```python
from build123d import *

# Parameters (mm, degrees)
SKETCH1_R           = 12.85
BOSS_EXTRUDE5_DEPTH = 10.58
SKETCH4_R           = 7.5
SKETCH4_R_2         = 4.5
BOSS_EXTRUDE6_DEPTH = 10.58


with BuildPart() as part:
    # Sketch1 → Boss-Extrude5 (new body)
    with BuildSketch(Plane.XY):
        Circle(SKETCH1_R)
    extrude(amount=BOSS_EXTRUDE5_DEPTH)

    # Sketch4 → Boss-Extrude6 (add)
    with BuildSketch(Plane(origin=(0, 0, 0), x_dir=(1, 0, 0), z_dir=(0, 1, 0))):
        with BuildLine():
            Line((-7.5, -10.58), (-7.5, -23.749253103))
            ThreePointArc((-7.5, -23.749253103), (0, -16.249253103), (7.5, -23.749253103))
            Line((7.5, -23.749253103), (7.5, -10.58))
            Line((7.5, -10.58), (-7.5, -10.58))
        make_face()
        with Locations((0, -23.749253103)):
            Circle(SKETCH4_R)
        with Locations((0, -23.749253103)):
            Circle(SKETCH4_R_2, mode=Mode.SUBTRACT)
        with Locations((0, -23.749253103)):
            Circle(SKETCH4_R_2)
    extrude(amount=BOSS_EXTRUDE6_DEPTH)


solid = part.part
```
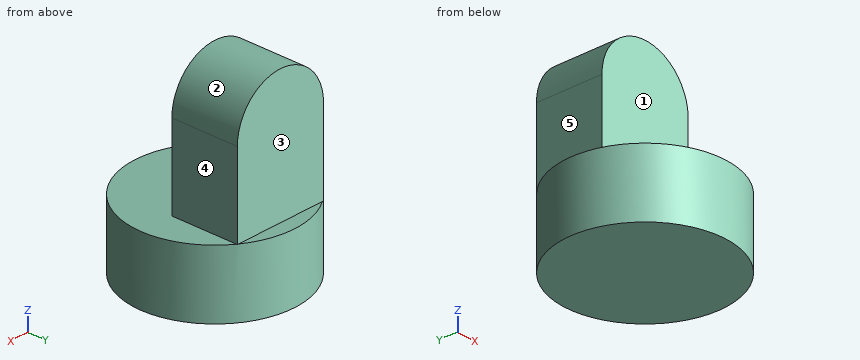
Model file for the job. Use its own axes, mm. Face numbers are marked on the shaded views. A direction names the side the tool comes from. Coordinates: 2 decimals unless noted, no trailing zeros. Write each loop counter-clockwise with the first axis right and the second up, starting at its lowest first coordinate (ties: lowest second). Pieces come first, ordered by that corner, then holes. Notation, with made-up numbers: (-6.5, 23) - (47.5, 23) arc R17 ccw to (47.5, 29) - close; hole circle Ø4 at (52.25, 83.25). An arc over 180 degrees is marked (long way). One line per question, with ' | ' between items. Start each with the question number.
Q1. Pin check, flat tips, straight feed: pin 1 (4 mm diameter, centred on y = 4, z = 14.5, fed in from -X); pin 2 (2 mm diameter, centred on x = 2.5, z = 11.5, fed in from -Y); pin 3 (6 mm diameter, centred on x = 2.5, z = 13.5, fed in from +Y); pin 4 (8 mm diameter, centred on y = -4.5, z = 20, fed in from -X). Stop position of each tip, or through.
Q2. 3-axis set-ups, long thin cutter, end or side, ignore diameter. For the marked faces 1, 2, 3, 4 and 5: which of +Z, -Z, +X, -X, +Y, -Y reach the whole face in a straight line?
Q3. Cut at B-B, the plane z = 19. List the corners of the cut face in (x, y), then the cut area to 3 significant figures.
Q4. Cut at D-D, the plane z = 6. List the corners of the cut face in (x, y), then the cut area to 3 significant figures.
Q5. Drill centre lines: line 1 (Y direction, x = 2.5, z = 27); line 2 (X direction, y = 0.25, z = 4.5). Where is each one in solid material? Low to high. Write a range as [from, to].
Q6. Cut at A-A, the plane x = 0. List the corners of the cut face in (y, z).
Q7. Cut at C-C, the plane y = 10. List the corners of the cut face in (x, z).
Answer below:
1) pin 1: x = -7.5 | pin 2: y = -12.68 | pin 3: y = 12.72 | pin 4: through
2) face 1: +Z, +X, -X, -Y | face 2: +Z, +Y, -Y | face 3: +Z, +X, -X, +Y | face 4: +Z, +X, +Y, -Y | face 5: +Z, -X, +Y, -Y
3) outline: (-7.5, 0) - (7.5, 0) - (7.5, 10.58) - (-7.5, 10.58) - close | area: 159 mm^2
4) outline: circle Ø25.7 at (0, 0) | area: 519 mm^2
5) line 1: [0, 10.58] | line 2: [-12.85, 12.85]
6) outline: (-12.85, 0) - (12.85, 0) - (12.85, 10.58) - (10.58, 10.58) - (10.58, 31.25) - (0, 31.25) - (0, 10.58) - (-12.85, 10.58) - close
7) outline: (-8.07, 0) - (8.07, 0) - (8.07, 10.58) - (7.5, 10.58) - (7.5, 23.75) arc R7.5 ccw to (-7.5, 23.75) - (-7.5, 10.58) - (-8.07, 10.58) - close
